Verification items for this drawing (mm, ordinates from the low corner). A direction names the side the tool comes from. Round coordinates to 2 decimals unless told otherwise and drop trailing zeros. Loops run counter-clockwise (first coordinate to the right, second up) from the corner with the lowest first, then second, coordinate; pieces in that order, holes last. Notation, with made-up numbers: (70, 84.25) - (86, 84.25) arc R22 cw to (86, 103.25) - close; hole circle Ø1 at (-13.75, 81.25). An arc over 180 degrees is marked (long way). Put each result on its own line as item: value.
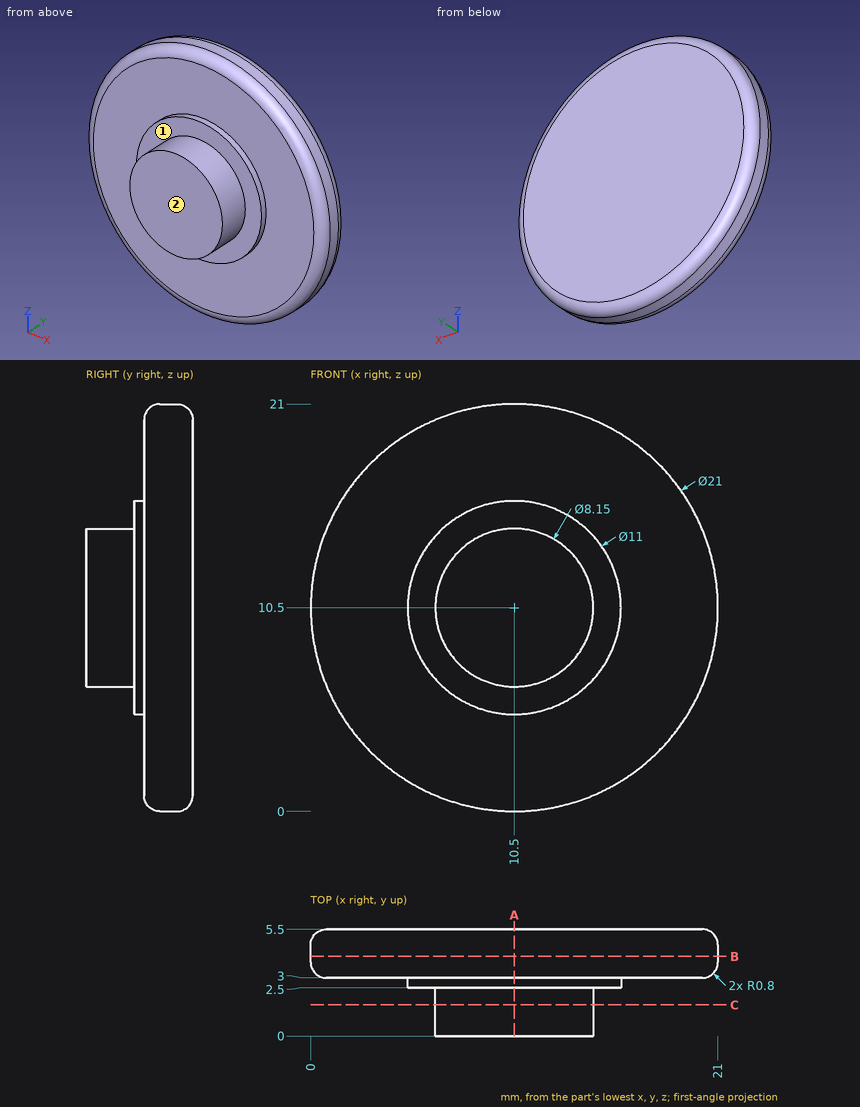
Item 1: Thickness scan on line 1 (Y direction, x = 18.25, z = 9.75); line 2 (Y direction, x = 14.75, z = 10); line 3 (Z direction, x = 12, y = 4.8). Record the ranges inside material, lowest first. Write a range as from..to.
Filled sheet:
line 1: 3..5.5
line 2: 2.5..5.5
line 3: 0.11..20.89
Item 2: Tool access check on the marked faces 1 and 2. Record the directions out of +Z, -Z, +X, -X, +Y, -Y that give a thin tool (end or side, any length) a straight path to the whole face; none if there is none.
Filled sheet:
face 1: -Y
face 2: +Z, -Z, +X, -X, -Y
Item 3: Section check C-C on y = 1.6. Enter the section's corners in (x, z) (3 decimals), then the cut area to 3 significant figures.
Filled sheet:
outline: circle Ø8.15 at (10.5, 10.5)
area: 52.2 mm²
Item 4: Go/stop test with flat-tipped pins: pin 1 (3 mm diameter, centred on x = 4.5, y = 4.5, fed in from +Z); pin 2 (6 mm diameter, centred on x = 13.5, z = 11, fed in from -Y); pin 3 (1.5 mm diameter, centred on y = 4.5, z = 17, fed in from +X); pin 4 (1.5 mm diameter, centred on y = 4.5, z = 5.5, fed in from -X). Record where each tip stops, or that it passes through.
Filled sheet:
pin 1: z = 19.99
pin 2: y = 0
pin 3: x = 19.29
pin 4: x = 0.9
Item 5: Section check A-A on x = 10.5. Enter the section's corners in (y, z) (3 decimals), then the cut area to 3 significant figures.
Filled sheet:
outline: (0, 6.425) - (2.5, 6.425) - (2.5, 5) - (3, 5) - (3, 0.8) arc R0.8 ccw to (3.8, 0) - (4.7, 0) arc R0.8 ccw to (5.5, 0.8) - (5.5, 20.2) arc R0.8 ccw to (4.7, 21) - (3.8, 21) arc R0.8 ccw to (3, 20.2) - (3, 16) - (2.5, 16) - (2.5, 14.575) - (0, 14.575) - close
area: 77.8 mm²
Item 6: Section check B-B on y = 4.1. Enter the section's corners in (x, z), then the cut area to 3 significant figures.
Filled sheet:
outline: circle Ø21 at (10.5, 10.5)
area: 346 mm²
